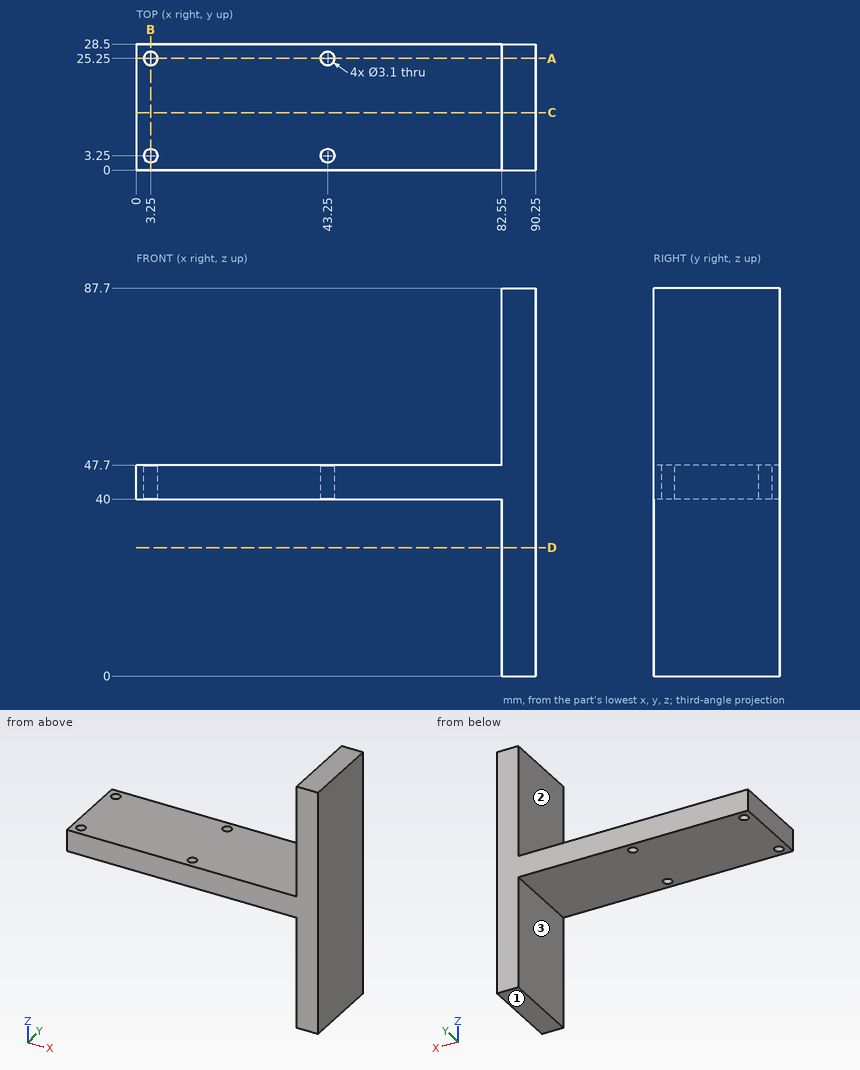
Part print with two shaded views. Sizes in mm from the minimum x, y, z corner. A direction names the side the tool comes from. Give positions to 0.01 mm unless a question says otherwise; leave off trailing zeros. Order: outer loops, then holes, each group sorted by start corner. A loop starts at its lowest first (then second) coordinate and runs counter-clockwise, first axis right, second up.
1) Saw through at B-B, the plane x = 3.25. Write the cut outline in (y, z), then the cut area to 3 significant figures.
2) Pin check, flat tips, straight feed: pin 1 (8.5 mm diameter, centred on y = 20, z = 15.5, fed in from -X); pin 2 (3.5 mm diameter, centred on x = 43.25, y = 3.25, fed in from +Z); pin 3 (8 mm diameter, centred on x = 46, y = 3.5, fed in from -Z). Stop position of each tip, or through.
3) Saw through at D-D, the plane z = 29. Write the cut outline in (x, y).
4) Wall check: probe 1 along Y at (x, z) = (3, 43); probe 2 along X at (y, z) = (3.25, 42); probe 3 along X at (y, z) = (8, 82). Give the ranges that are in metal, low to high.
5) 3-axis set-ups, long thin cutter, end or side, ignore diameter. For the marked faces 1, 2 and 3: which of +Z, -Z, +X, -X, +Y, -Y reach the whole face in a straight line?
6) Saw through at C-C, the plane y = 13. Write the cut outline in (x, z), then the cut area to 3 significant figures.
7) Saw through at A-A, the plane y = 25.25. Write the cut outline in (x, z).
Computed:
1. outline: (0, 40) - (1.7, 40) - (1.7, 47.7) - (0, 47.7) - close; (4.8, 40) - (23.7, 40) - (23.7, 47.7) - (4.8, 47.7) - close; (26.8, 40) - (28.5, 40) - (28.5, 47.7) - (26.8, 47.7) - close
1. area: 172 mm2
2. pin 1: stops at x = 82.55
2. pin 2: stops at z = 47.7
2. pin 3: stops at z = 40
3. outline: (82.55, 0) - (90.25, 0) - (90.25, 28.5) - (82.55, 28.5) - close
4. probe 1: y = 0 to 1.72, 4.78 to 23.72, 26.78 to 28.5
4. probe 2: x = 0 to 1.7, 4.8 to 41.7, 44.8 to 90.25
4. probe 3: x = 82.55 to 90.25
5. face 1: -Z, +X, -X, +Y, -Y
5. face 2: +Z, -X, +Y, -Y
5. face 3: -Z, -X, +Y, -Y
6. outline: (0, 40) - (82.55, 40) - (82.55, 0) - (90.25, 0) - (90.25, 87.7) - (82.55, 87.7) - (82.55, 47.7) - (0, 47.7) - close
6. area: 1,310 mm2
7. outline: (0, 40) - (1.7, 40) - (1.7, 47.7) - (0, 47.7) - close; (4.8, 40) - (41.7, 40) - (41.7, 47.7) - (4.8, 47.7) - close; (44.8, 40) - (82.55, 40) - (82.55, 0) - (90.25, 0) - (90.25, 87.7) - (82.55, 87.7) - (82.55, 47.7) - (44.8, 47.7) - close
